from build123d import *

# Parameters (mm, degrees)
ESTRUSIONE_ESTRUSIONE1_DEPTH      = 5
ESTRUSIONE_ESTRUSIONE1_DEPTH_BACK = 2
SCHIZZO4_R                        = 4.5
ESTRUSIONE_ESTRUSIONE3_DEPTH      = 8
SCHIZZO5_W                        = 10
SCHIZZO5_H                        = 10
TAGLIO_ESTRUSIONE1_DEPTH          = 6
SCHIZZO6_W                        = 5.883874728
SCHIZZO6_H                        = 31.765714376
TAGLIO_ESTRUSIONE3_DEPTH          = 15
TAGLIO_ESTRUSIONE3_DEPTH_BACK     = 15
SCHIZZO7_R                        = 4.5
TAGLIO_ESTRUSIONE4_DEPTH          = 3


with BuildPart() as part:
    # Schizzo1 → Estrusione-Estrusione1 (new body, two sides)
    with BuildSketch(Plane.XY) as estrusione_estrusione1_sk:
        with BuildLine():
            Line((-19.735743023, 33.889071348), (-19.735743023, 43.889071348))
            ThreePointArc((-19.735743023, 43.889071348), (-12.529677135, 46.069061439), (-5.323611247, 43.889071348))
            Line((-5.323611247, 43.889071348), (-5.323611247, 33.889071348))
            ThreePointArc((-5.323611247, 33.889071348), (-7.707011318, 29.345426307), (-8.529677135, 24.280988816))
            Line((-8.529677135, 24.280988816), (-8.529677135, 2.230988816))
            ThreePointArc((-8.529677135, 2.230988816), (-12.529677135, -16.934162574), (-16.529677135, 2.230988816))
            Line((-16.529677135, 2.230988816), (-16.529677135, 24.280988816))
            ThreePointArc((-16.529677135, 24.280988816), (-17.352342952, 29.345426307), (-19.735743023, 33.889071348))
        make_face()
    extrude(amount=ESTRUSIONE_ESTRUSIONE1_DEPTH)
    extrude(estrusione_estrusione1_sk.sketch, amount=-ESTRUSIONE_ESTRUSIONE1_DEPTH_BACK)

    # Schizzo4 → Estrusione-Estrusione3 (add)
    with BuildSketch(Plane.XY.offset(5)):
        with Locations((-12.529677135, 38.889071348)):
            Circle(SCHIZZO4_R)
    extrude(amount=ESTRUSIONE_ESTRUSIONE3_DEPTH)

    # Schizzo5 → Taglio-Estrusione1 (cut)
    with BuildSketch(Plane(origin=(0, 0, -2), x_dir=(-1, 0, 0), z_dir=(0, 0, -1))):
        with Locations((12.529677135, -6.934162574)):
            Rectangle(SCHIZZO5_W, SCHIZZO5_H)
    extrude(amount=-TAGLIO_ESTRUSIONE1_DEPTH, mode=Mode.SUBTRACT)

    # Schizzo6 → Taglio-Estrusione3 (cut, two sides)
    with BuildSketch(Plane.ZY.offset(16.529677135)) as taglio_estrusione3_sk:
        with Locations((4.941937364, 18.113846004)):
            Rectangle(SCHIZZO6_W, SCHIZZO6_H)
    extrude(amount=TAGLIO_ESTRUSIONE3_DEPTH, mode=Mode.SUBTRACT)
    extrude(taglio_estrusione3_sk.sketch, amount=-TAGLIO_ESTRUSIONE3_DEPTH_BACK, mode=Mode.SUBTRACT)

    # Schizzo7 → Taglio-Estrusione4 (cut)
    with BuildSketch(Plane.XY.offset(5)):
        Polygon((-26.342217031, 45.266793591), (-24.610237107, 33.489330106), (-19.735743023, 33.889071348), (-1.055310137, 33.889071348), (-1.98835975, 45.266793591), (-13.868873062, 49.75887888), align=None)
        with Locations((-12.529677135, 38.889071348)):
            Circle(SCHIZZO7_R, mode=Mode.SUBTRACT)
    extrude(amount=-TAGLIO_ESTRUSIONE4_DEPTH, mode=Mode.SUBTRACT)


solid = part.part
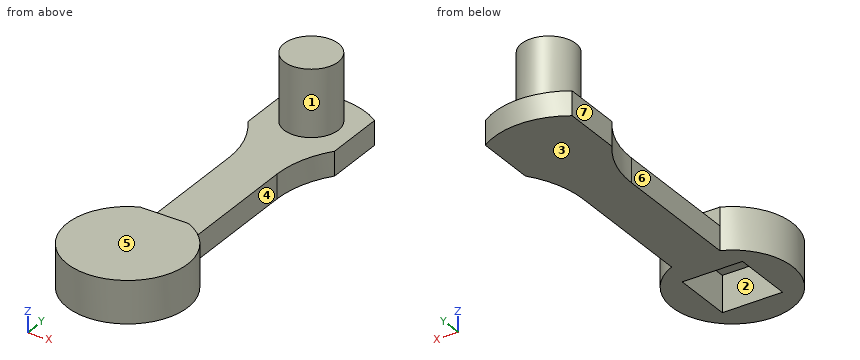
The listing builds one solid part. Answer for the finished solid, in the listing's coordinates (mm). Face numbers are marked on the shaded views. A direction names the side the tool comes from. Round coordinates to 2 decimals unless told otherwise and drop trailing zeros. Order: outer loops, then holes, each group sorted by start corner. A loop starts at its lowest first (then second) coordinate and runs counter-clockwise, first axis right, second up. Notation, with made-up numbers: (62.5, 85.25) - (115.5, 85.25) arc R29 ccw to (115.5, 119.25) - close; hole circle Ø5 at (-8.5, -34). An arc over 180 degrees is marked (long way). Write item = value, one per line. Start each with the question number.
1) Section B-B, the plane x = -18.75 is taken. Write down the section's boundary in (y, z), plus the area to 3 significant figures.
2) Section D-D, the plane x = -9.75 is taken. Write down the section's boundary in (y, z), plus the area to 3 significant figures.
3) For the marked faces 4, 5, 6 and 7, determine the directions among +Z, -Z, +X, -X, +Y, -Y from which every point of the face is accessible in a straight line to the end or side of a thin tool.
4) Given pin 1 (3 mm diameter, centred on y = 37.5, z = 1, fed in from -X); pin 2 (1.5 mm diameter, centred on x = -12, z = 4, fed in from +Y); pin 3 (8 mm diameter, centred on x = -5, y = 34, fed in from +Z); pin 4 (1.5 mm diameter, centred on x = -18, y = 19, fed in from -Z), each flat-ended and moving along its own axis, determine where each tip first touches the part or whether it passes through.
5) Section C-C, the plane y = -10.5 is taken. Write down the section's boundary in (x, z), plus the area to 3 significant figures.
6) Section A-A, the plane z = 3.25 is taken. Write down the section's boundary in (x, y).
7) Straight lines are drawn through the part: L1, parallel to Y at x = -14.5, z = 2.5; L2, parallel to Z at x = -12.5, y = 10; L3, parallel to X at y = 24, z = 1.75. For each, find the intervals that lie inside material, in ascending order.
8) For a pull along X with two mould halves and no side action, classify the marked faces 1, 2 and 3 as released by +X, released by -X, zero draft, split by the parting line, or undercut.
Results list:
q1.outline = (-14.76, -2) - (0.9, -2) - (0.9, 5) - (-14.76, 5) - close; (32.41, -2) - (44.48, -2) - (44.48, 2) - (32.41, 2) - close
q1.area = 158 mm^2
q2.outline = (-16.54, -2) - (-11.93, -2) - (-11.93, 4) - (-1.93, 4) - (-1.93, -2) - (45.77, -2) - (45.77, 2) - (42.43, 2) - (42.43, 13) - (35.35, 13) - (35.35, 2) - (2.23, 2) - (2.23, 5) - (-16.54, 5) - close
q2.area = 323 mm^2
q3.face_4 = +Z, -Z, +X
q3.face_5 = +Z, +X, -X, -Y
q3.face_6 = +Z, -Z, -X
q3.face_7 = +Z, -Z, -X, +Y
q4.pin_1 = -19.74
q4.pin_2 = 43.39
q4.pin_3 = 2
q4.pin_4 = through
q5.outline = (-21.87, -2) - (-17.53, -2) - (-17.53, 4) - (-7.53, 4) - (-7.53, -2) - (-3.19, -2) - (-3.19, 5) - (-21.87, 5) - close
q5.area = 70.8 mm^2
q6.outline = circle Ø9 at (-12.53, 38.89); (-16.53, 2.23) arc R10 ccw (long way) to (-8.53, 2.23) - close; hole (-17.53, -11.93) - (-7.53, -11.93) - (-7.53, -1.93) - (-17.53, -1.93) - close
q7.L1 = -16.74 to -11.93, -1.93 to 2.23, 34.84 to 42.93
q7.L2 = -2 to 2
q7.L3 = -16.53 to -8.53
q8.face_1 = split by the parting line
q8.face_2 = undercut
q8.face_3 = zero draft
